Can you work these out from the model? Positions are in its coordinate system, mm. Face numbers are marked on the shaded views. A direction names the side the tool comes from. Coordinates: 2 decimals unless noted, no trailing zeros. Write each loop counter-clockwise with the first axis right and the second up, starting at its lowest first coordinate (ties: lowest second). Pieces come first, ordered by that corner, then holes. Notation, with made-up numbers: M -32.75,-29.75 L 9.25,-29.75 A25 ccw 9.25,-9.75 Z; hole C 49.25,-32 d5. An arc over 180 degrees is marked long. Use one line per item in the form item = value. Start each with the question number.
```python
from build123d import *

# Parameters (mm, degrees)
CYLINDER003_R     = 3
CYLINDER003_DEPTH = 10
ARRAY_COUNT       = 8
CYLINDER002_R     = 10
CYLINDER002_DEPTH = 30
CYLINDER001_R     = 15
CYLINDER001_DEPTH = 12
CYLINDER_R        = 30
CYLINDER_DEPTH    = 5


with BuildPart() as array:
    # Cylinder003 → Cylinder003 (new body)
    with BuildSketch(Plane(origin=(22, 0, 0), x_dir=(1, 0, 0), z_dir=(0, 0, 1))):
        Circle(CYLINDER003_R)
    extrude(amount=CYLINDER003_DEPTH)

    # Array: Array ×8 about axis
    array_axis = Axis((0, 0, 0), (0, 0, 1))


with BuildPart() as array_1:
    add(array.part)
    for i in range(1, ARRAY_COUNT):
        add(array.part.rotate(array_axis, i * 360 / ARRAY_COUNT))


with BuildPart() as array_2:
    # Array placement: moved
    add(array_1.part.moved(Location((0, 0, -1))))


with BuildPart() as tubo_interior:
    # Cylinder002 → Cylinder002 (new body)
    with BuildSketch(Plane.XY.offset(-1)):
        Circle(CYLINDER002_R)
    extrude(amount=CYLINDER002_DEPTH)


with BuildPart() as tubo_exterior:
    # Cylinder001 → Cylinder001 (new body)
    with BuildSketch(Plane.XY.offset(-1)):
        Circle(CYLINDER001_R)
    extrude(amount=CYLINDER001_DEPTH)


with BuildPart() as cut001:
    # Cylinder → Cylinder (new body)
    with BuildSketch(Plane.XY):
        Circle(CYLINDER_R)
    extrude(amount=CYLINDER_DEPTH)

    # Fusion: union tubo_exterior
    add(tubo_exterior.part)

    # Cut: cut tubo_interior
    add(tubo_interior.part, mode=Mode.SUBTRACT)

    # Cut001: cut Array
    add(array_2.part, mode=Mode.SUBTRACT)


solid = cut001.part
```
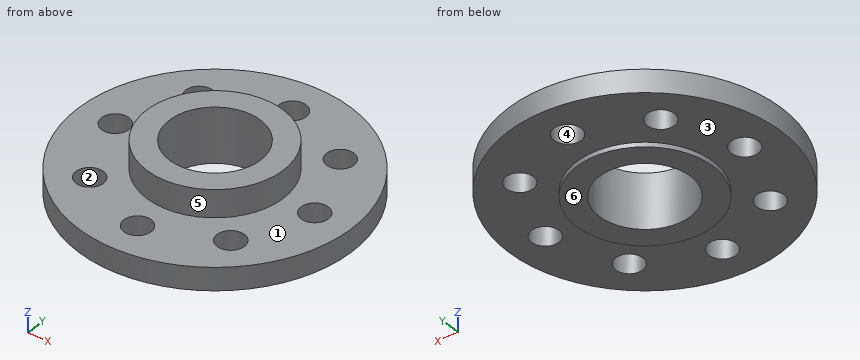
1) Suppose I cut it at C-C on y = -22.5. Please give me the cut outline in (x, z).
2) If we mould it in two halves opening along X, with no side actions, what happens to the marked faces 4, 5 and 6? For each: +X half, -X half, draft (parallel to the pull), parting line (faces both ways), or undercut.
3) Which directions (+Z, -Z, +X, -X, +Y, -Y) give clear straight access to the entire face, cutting with the end or side of a thin tool? Please do the marked faces 1, 2 and 3.
4) Suppose I cut it at A-A on y = 0. Please give me the cut outline in (x, z), and give its area (3 significant figures).
5) Suppose I cut it at D-D on z = 1. State how many separate pieces and enclosed holes the cut face has, and give its area (3 significant figures).
6) Please list where these lines run through material, in increasing order: line 1 (Y direction, x = 1, z = 1.75); line 2 (Z direction, x = 26, y = 2); line 3 (Y direction, x = -5, z = 7).
7) Will these pins go through, and if not, where does the flat tip stop? pin 1 Ø7 at (x, y) = (0, 22) entering from +Z; pin 2 Ø5 at (x, y) = (-15.56, -15.56) entering from +Z; pin 3 Ø2 at (x, y) = (-17, 13.5) entering from -Z; pin 4 Ø5 at (x, z) = (3, 1.5) entering from +Y.
Computed values:
q1.outline = M -19.84,0 L -2.96,0 L -2.96,5 L -19.84,5 Z; M 2.96,0 L 19.84,0 L 19.84,5 L 2.96,5 Z
q2.face_4 = undercut
q2.face_5 = parting line
q2.face_6 = draft
q3.face_1 = +Z
q3.face_2 = +Z, -Z
q3.face_3 = -Z
q4.outline = M -30,0 L -25,0 L -25,5 L -30,5 Z; M -19,0 L -15,0 L -15,-1 L -10,-1 L -10,11 L -15,11 L -15,5 L -19,5 Z; M 10,-1 L 15,-1 L 15,0 L 19,0 L 19,5 L 15,5 L 15,11 L 10,11 Z; M 25,0 L 30,0 L 30,5 L 25,5 Z
q4.area = 210 mm²
q5.separate_pieces = 1
q5.enclosed_holes = 9
q5.area = 2,290 mm²
q6.line_1 = -29.98 to -24.83, -19.17 to -9.95, 9.95 to 19.17, 24.83 to 29.98
q6.line_2 = 0 to 5
q6.line_3 = -14.14 to -8.66, 8.66 to 14.14
q7.pin_1 = 5
q7.pin_2 = through
q7.pin_3 = 0
q7.pin_4 = 30
